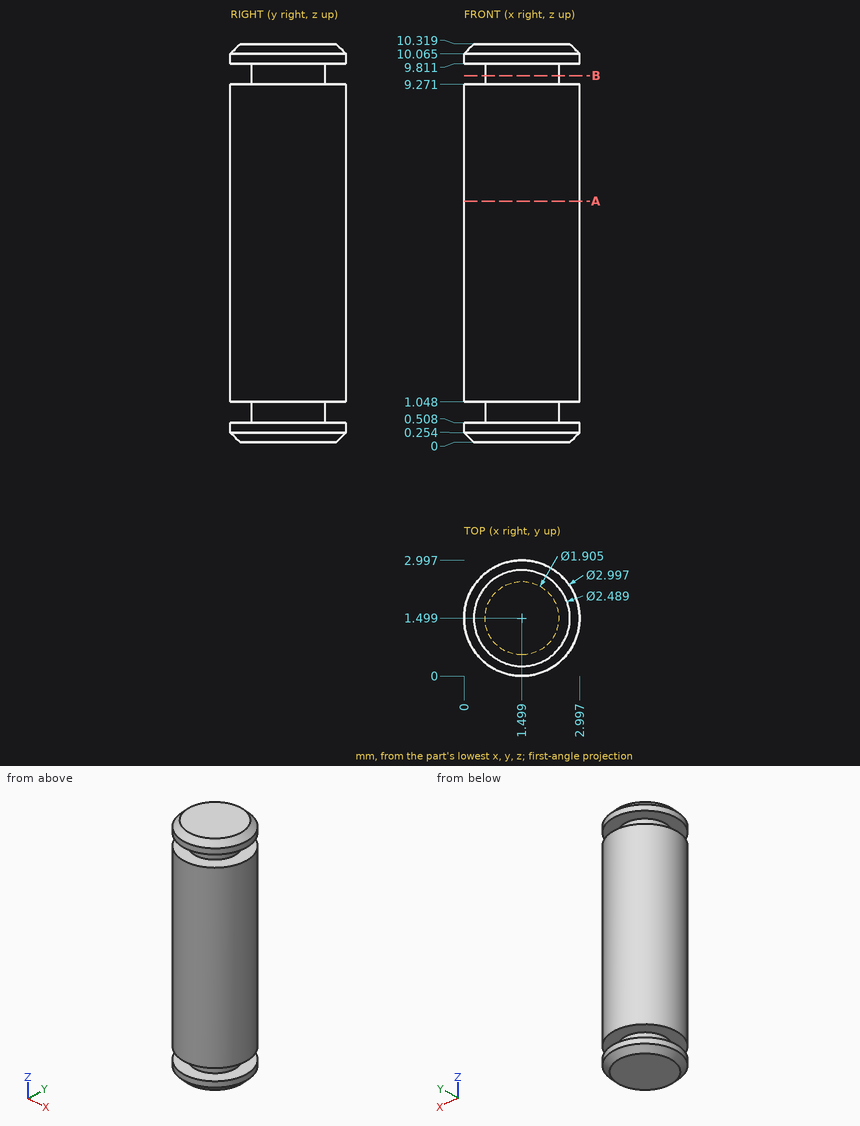
Study the drawing (mm; zero at the part's minimum x, y, z) and answer. Round coordinates to 2 decimals unless told otherwise and drop trailing zeros. Order: outer loops, then holes, each group sorted by start corner. A loop starts at its lowest first (then second) coordinate and runs counter-clockwise, first axis right, second up. Notation, with made-up numbers: (70.5, -28) -> (89.5, -28) arc R30 ccw to (89.5, -5) -> close; hole circle Ø4 at (46.25, 46.25). An arc over 180 degrees is marked (long way). Answer as CSV lines item,"result". Start each with the question number.
(1) The part is cut by section A-A (z = 6.25). Determine the outline of the cut face in (x, y).
(2) The part is cut by section B-B (z = 9.5). Determine the outline of the cut face in (x, y) (1 decimal).
(3) Find the intervals of material crossed by probe 1 along Z at (x, y) = (0.65, 0.7); probe 2 along Z at (x, y) = (0.15, 1.95); probe 3 along Y at (x, z) = (1.3, 2.75) (1 decimal), in increasing order. Write a range as from..to.
(4) Flat-ended cylindrical pins translate along their axes: pin 1 Ø1.5 at (x, z) = (2.5, 8.5) entering from +Y; pin 2 Ø1.5 at (x, z) = (2.5, 8) entering from -Y. Find the tip coordinate at first contact, or state that the pin passes through.
Evaluation:
1,outline,"circle Ø3 at (1.5, 1.5)"
2,outline,"circle Ø1.9 at (1.5, 1.5)"
3,probe 1,"0..0.51, 1.05..9.27, 9.81..10.32"
3,probe 2,"0.18..0.51, 1.05..9.27, 9.81..10.14"
3,probe 3,"0..3"
4,pin 1,"y = 2.98"
4,pin 2,"y = 0.02"
